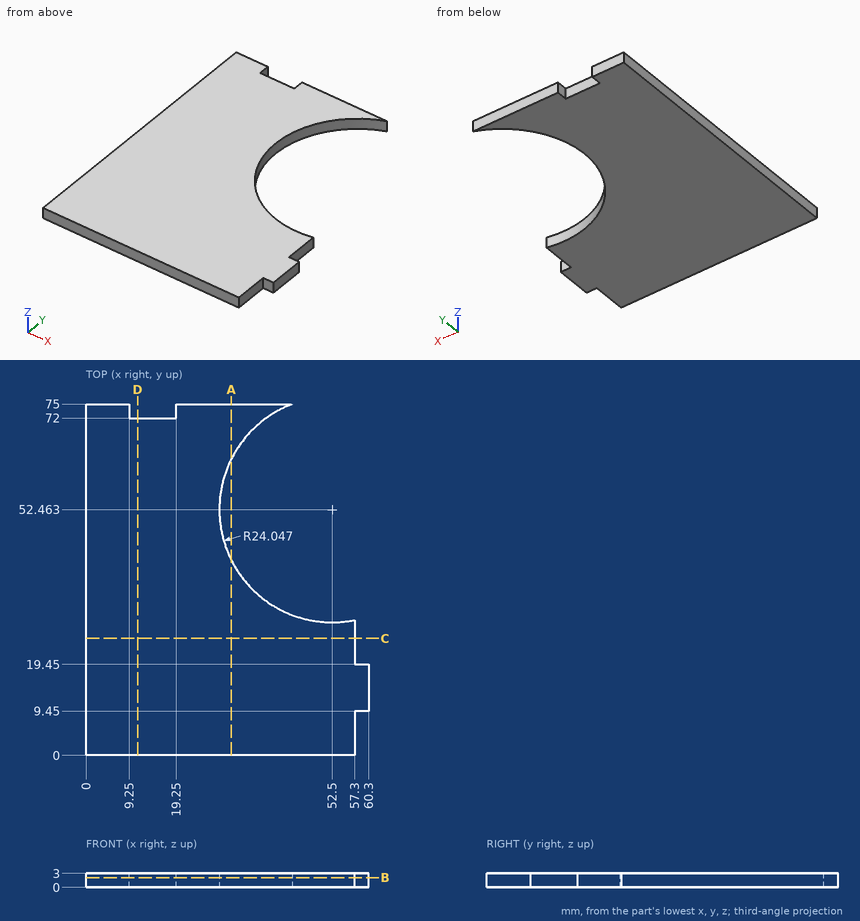
Design review of the part shown in the three views and the two pictorial views. Dimensions are in mm from the part's minimum x, y and z. Round coordinates to 2 decimals unless told otherwise and drop trailing zeros. Write each loop counter-clockwise with the first axis right and the second up, starting at its lowest first coordinate (ties: lowest second). Pieces come first, ordered by that corner, then holes. Notation, with made-up numbers: (66, 43) -> (94, 43) arc R15 ccw to (94, 53) -> close; hole circle Ø8 at (-18, -21). An arc over 180 degrees is marked (long way). Write item = value, one per line. Start each with the question number.
1) Clearance check with flat-ended pins moving along their axes: pin 1 (1.5 mm diameter, centred on y = 22, z = 1.5, fed in from +X); pin 2 (1.5 mm diameter, centred on x = 13, z = 0.5, fed in from +Y); pin 3 (1.5 mm diameter, centred on x = 58.5, z = 2, fed in from -Y). State where each tip first meets the part, or that it passes through.
2) Take a section at A-A, the plane x = 31. State the section outline as (y, z) points, plus the area to 3 significant figures.
3) Take a section at D-D, the plane x = 11. State the section outline as (y, z) points.
4) Take a section at B-B, the plane z = 2.1. State the section outline as (x, y) points, plus the area to 3 significant figures.
5) Take a section at C-C, the plane y = 25. State the section outline as (x, z) points, plus the area to 3 significant figures.
6) Wall thickness on probe 1 along Y at (x, z) = (13.5, 0.7); probe 2 along Y at (x, z) = (40.5, 2.15) (1 decimal); probe 3 along X at (y, z) = (27, 1): over which ranges is each line inside the solid? List them lowest first. Write a range as from..to.
Results list:
q1.pin_1 = 57.3
q1.pin_2 = 72
q1.pin_3 = 9.45
q2.outline = (0, 0) -> (41.69, 0) -> (41.69, 3) -> (0, 3) -> close; (63.23, 0) -> (75, 0) -> (75, 3) -> (63.23, 3) -> close
q2.area = 160 mm²
q3.outline = (0, 0) -> (72, 0) -> (72, 3) -> (0, 3) -> close
q4.outline = (0, 0) -> (57.3, 0) -> (57.3, 9.45) -> (60.3, 9.45) -> (60.3, 19.45) -> (57.3, 19.45) -> (57.3, 28.9) arc R24.05 cw to (44.11, 75) -> (19.25, 75) -> (19.25, 72) -> (9.25, 72) -> (9.25, 75) -> (0, 75) -> close
q4.area = 3,170 mm²
q5.outline = (0, 0) -> (57.3, 0) -> (57.3, 3) -> (0, 3) -> close
q5.area = 172 mm²
q6.probe_1 = 0..72
q6.probe_2 = 0..31.6, 73.3..75
q6.probe_3 = 0..57.3
